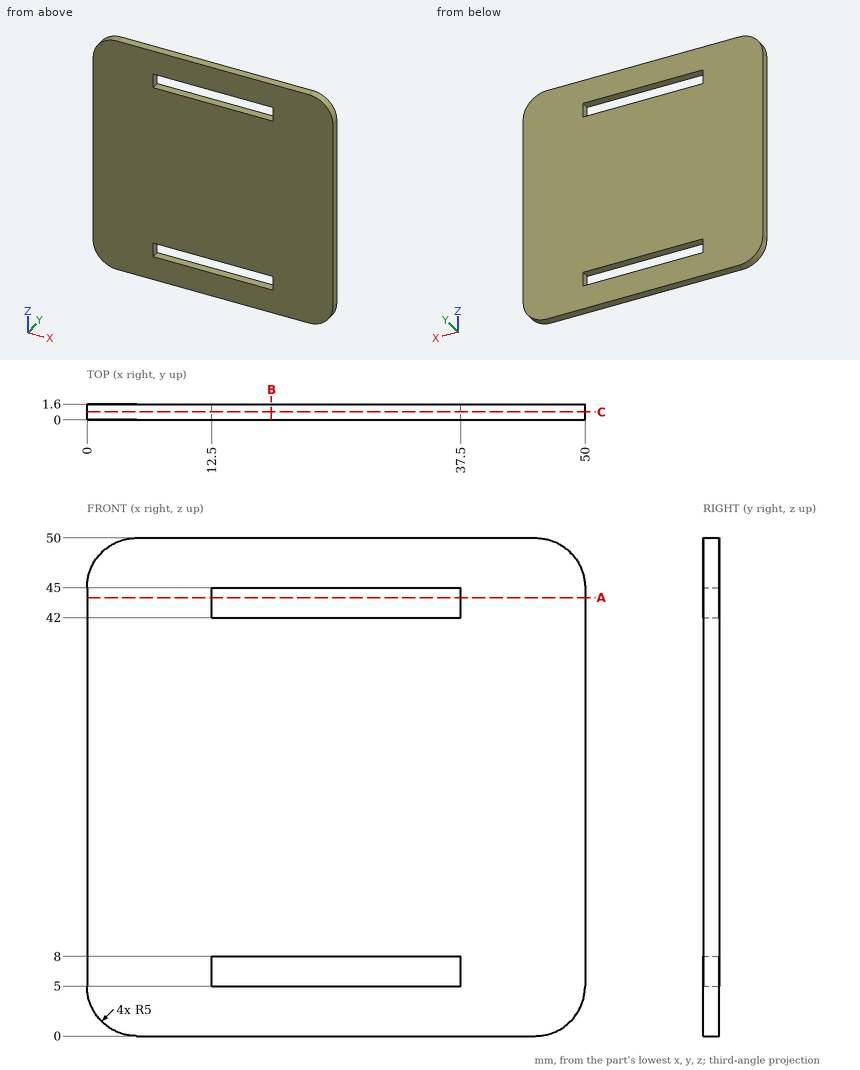
Geometry: see drawing. Coordinates: mm, zero at the bounding-box minimum. Round coordinates to 2 decimals unless told otherwise and drop trailing zeros. Write each loop counter-clockwise with the first axis right and the second up, starting at its lowest first coordinate (ties: lowest second). Pieces come first, ordered by that corner, then holes. Notation, with made-up numbers: (43, 55) -> (92, 55) arc R23 ccw to (92, 72) -> close; hole circle Ø10 at (46, -33.5). An arc over 180 degrees is marked (long way). Answer as CSV lines item,"result".
1. Section C-C (y = 0.8). Return the cut outline in (x, z), plus the area to 3 significant figures.
Geometry says:
outline,"(0, 5) arc R5 ccw to (5, 0) -> (45, 0) arc R5 ccw to (50, 5) -> (50, 45) arc R5 ccw to (45, 50) -> (5, 50) arc R5 ccw to (0, 45) -> close; hole (12.5, 5) -> (37.5, 5) -> (37.5, 8) -> (12.5, 8) -> close; hole (12.5, 42) -> (37.5, 42) -> (37.5, 45) -> (12.5, 45) -> close"
area,"2,330 mm^2"
2. Section B-B (x = 18.5). Return the cut outline in (y, z).
Geometry says:
outline,"(0, 0) -> (1.6, 0) -> (1.6, 5) -> (0, 5) -> close; (0, 8) -> (1.6, 8) -> (1.6, 42) -> (0, 42) -> close; (0, 45) -> (1.6, 45) -> (1.6, 50) -> (0, 50) -> close"
3. Ray query, L1, parallel to Z at x = 21, y = 1.25; L2, parallel to X at y = 1, z = 44; L3, parallel to Z at x = 3.5, y = 1.35. Return the intervals inside material, ascending. Write a range as [from, to].
Geometry says:
L1,"z = [0, 5], [8, 42], [45, 50]"
L2,"x = [0, 12.5], [37.5, 50]"
L3,"z = [0.23, 49.77]"
4. Section A-A (z = 44). Return the cut outline in (x, y), plus the area to 3 significant figures.
Geometry says:
outline,"(0, 0) -> (12.5, 0) -> (12.5, 1.6) -> (0, 1.6) -> close; (37.5, 0) -> (50, 0) -> (50, 1.6) -> (37.5, 1.6) -> close"
area,"40.0 mm^2"
